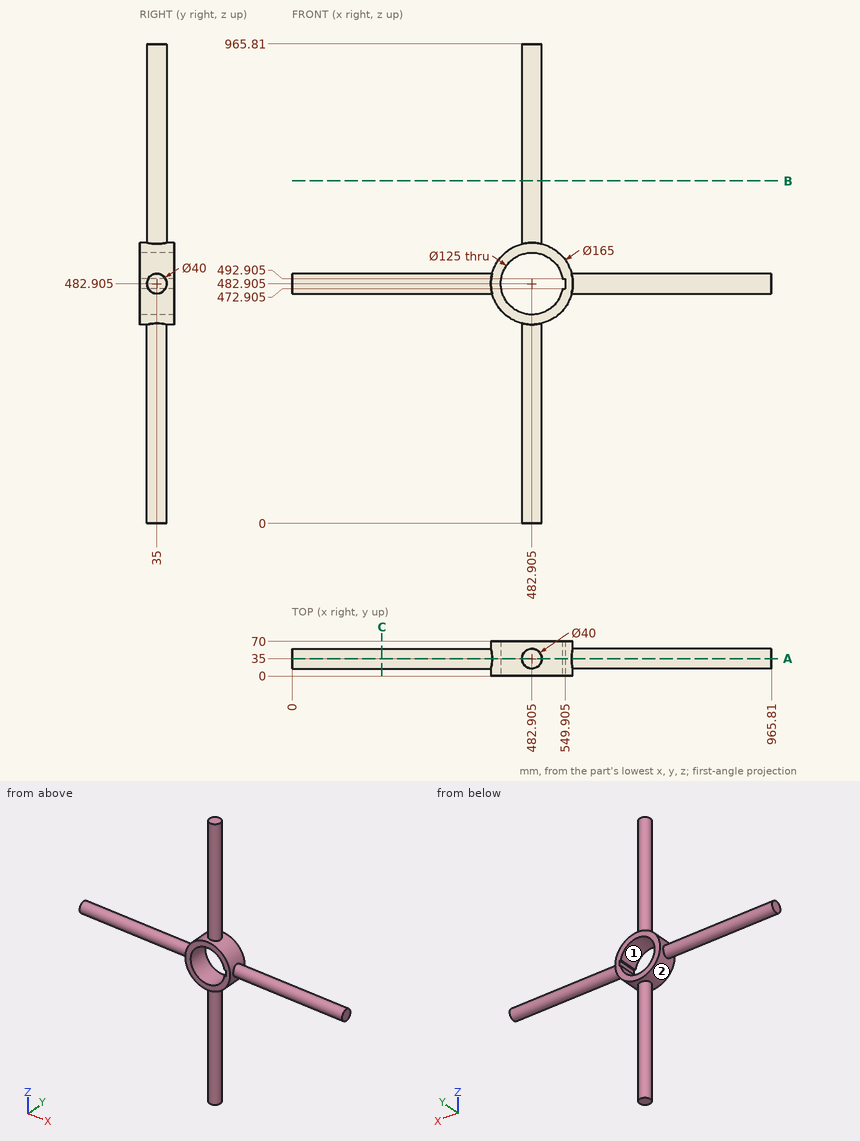
Part print with two shaded views. Sizes in mm from the minimum x, y, z corner. Coordinates: 2 decimals unless noted, no trailing zeros. Order: outer loops, then holes, each group sorted by start corner. A loop starts at its lowest first (then second) coordinate and runs counter-clockwise, first axis right, second up. Notation, with made-up numbers: (57, 7.25) - (74, 7.25) arc R23 ccw to (74, 21.25) - close; hole circle Ø8 at (60.5, 30.25). An arc over 180 degrees is marked (long way). Write item = value, one per line. Start each with the question number.
1) Flat gauge pins, fed straight in: pin 1 Ø4 at (y, z) = (40.5, 186) entering from -X; pin 2 Ø4 at (y, z) = (31.5, 542.5) entering from +X; pin 3 Ø1.5 at (x, y) = (324, 13.5) entering from -Z; pin 4 Ø1.6 at (x, y) = (546.5, 39.5) entering from +Z. Where does each tip first touch, or does it go through?
2) Two-plate mould, pull along Z, no slides. Class the marked faces 1 and 2: pulls with the +Z half, pulls with the -Z half, needs draft (parallel to the pull), parting line crosses it, or undercut.
3) Saw through at A-A on y = 35. Write the cut outline in (x, z) (1 decimal).
4) Saw through at C-C on x = 180.5. Write the cut outline in (y, z) (1 decimal).
5) Saw through at B-B on z = 690. Write the cut outline in (x, y) (1 decimal), then the cut area to 3 significant figures.
6) Wall check: line 1 along X through (y, z) = (36, 103.5); line 2 along Z through (x, y) = (350.5, 26) (1 decimal); line 3 along Y through (x, z) = (127, 488.5). Give the ranges that are in metal, low to high. Write a range as from..to.
From the geometry:
q1.pin_1 = 463.21
q1.pin_2 = 541.97
q1.pin_3 = through
q1.pin_4 = 536.41
q2.face_1 = undercut
q2.face_2 = parting line crosses it
q3.outline = (0, 462.9) - (402.9, 462.9) arc R82.5 ccw to (462.9, 402.9) - (462.9, 0) - (502.9, 0) - (502.9, 402.9) arc R82.5 ccw to (562.9, 462.9) - (965.8, 462.9) - (965.8, 502.9) - (562.9, 502.9) arc R82.5 ccw to (502.9, 562.9) - (502.9, 965.8) - (462.9, 965.8) - (462.9, 562.9) arc R82.5 ccw to (402.9, 502.9) - (0, 502.9) - close; hole (544.6, 472.9) - (549.9, 472.9) - (549.9, 492.9) - (544.6, 492.9) arc R62.5 ccw (long way) to start
q4.outline = circle Ø40 at (35, 482.9)
q5.outline = circle Ø40 at (482.9, 35)
q5.area = 1,260 mm^2
q6.line_1 = 462.93..502.88
q6.line_2 = 465..500.8
q6.line_3 = 15.8..54.2
